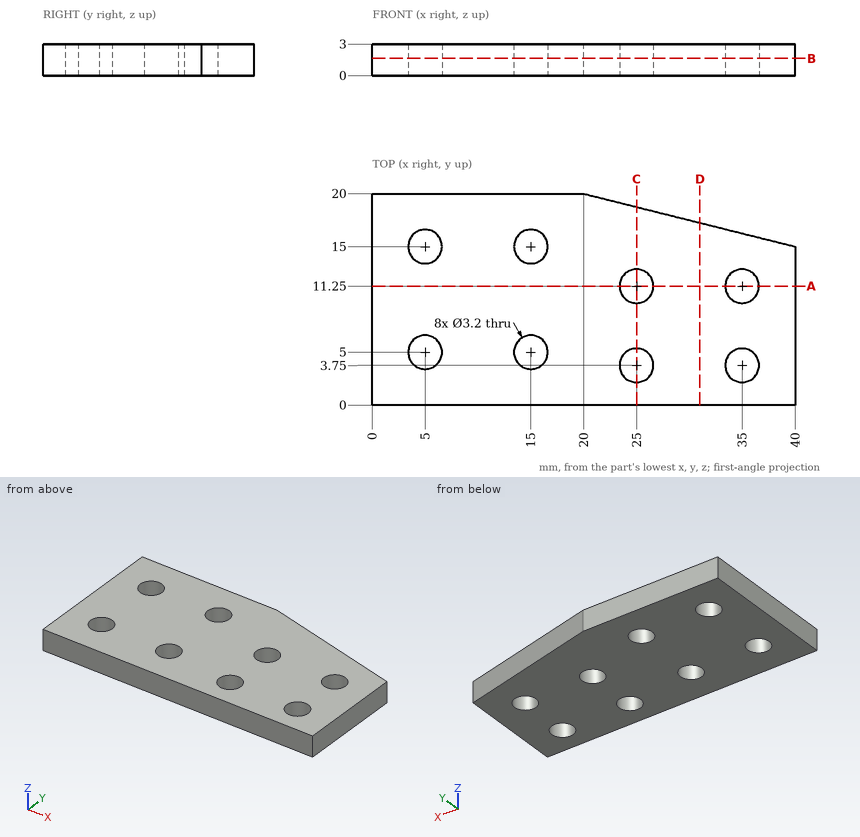
Answer from the drawing. Dimensions are ordinates in mm from the lowest x, y and z of the part. Give positions to 0.01 mm unless a question says otherwise; leave off trailing zeros. Loops run counter-clockwise (first coordinate to the right, second up) from the corner with the lowest first, then second, coordinate; pieces in that order, holes last.
Item 1: A cutting plane is placed at D-D (x = 31). Give the vertices of the cut face in (y, z), then the cut area to 4 significant figures.
Derived:
outline: (0, 0) - (17.25, 0) - (17.25, 3) - (0, 3) - close
area: 51.75 mm2
Item 2: A cutting plane is placed at B-B (z = 1.65). Give the number of separate pieces and of enclosed holes in the cut face, then the cut area to 3 significant figures.
Derived:
separate pieces: 1
enclosed holes: 8
area: 686 mm2
Item 3: Find the intervals of material crossed by line 1 along Y through (x, z) = (5, 0.95); line 2 along X through (y, z) = (5.5, 0.75); line 3 along Y through (x, z) = (25, 0.4), in increasing order.
Derived:
line 1: y = 0 to 3.4, 6.6 to 13.4, 16.6 to 20
line 2: x = 0 to 3.48, 6.52 to 13.48, 16.52 to 40
line 3: y = 0 to 2.15, 5.35 to 9.65, 12.85 to 18.75
Item 4: A cutting plane is placed at A-A (y = 11.25). Give the vertices of the cut face in (x, z).
Derived:
outline: (0, 0) - (23.4, 0) - (23.4, 3) - (0, 3) - close; (26.6, 0) - (33.4, 0) - (33.4, 3) - (26.6, 3) - close; (36.6, 0) - (40, 0) - (40, 3) - (36.6, 3) - close
Item 5: A cutting plane is placed at C-C (x = 25). Give the vertices of the cut face in (y, z), then the cut area to 4 significant figures.
Derived:
outline: (0, 0) - (2.15, 0) - (2.15, 3) - (0, 3) - close; (5.35, 0) - (9.65, 0) - (9.65, 3) - (5.35, 3) - close; (12.85, 0) - (18.75, 0) - (18.75, 3) - (12.85, 3) - close
area: 37.05 mm2
